Autodesk Inventor part; units mm, degrees
ref_plane "Work Plane2" through (-73.7, 7.425, 1.675) normal (-1, 0, 0) x (0, 0, 1)
ref_plane "Work Plane4" through (-27.2, 7.425, 1.675) normal (1, 0, 0) x (0, 1, 0)
ref_plane "Work Plane6" through (-32.2, 6.75, 1) normal (1, 0, 0) x (0, 1, 0)
ref_plane "Work Plane1" through (-24.5, 21.125, 15.375) normal (1, 0, 0) x (0, -1, 0)
sketch "Sketch1" plane through (-24.5, 21.125, 15.375) normal (1, 0, 0) x (0, -1, 0)
  line L0 (-16.375, 15.375) -> (19, 15.375)
  line L1 (19, 15.375) -> (19, -3.0564)
  line L2 (19, -3.0564) -> (-16.375, -3.0564)
  line L3 (-16.375, -3.0564) -> (-16.375, 15.375)
  circle A0 centre (1, 0) radius 5
  circle A1 centre (9, 0) radius 1.0564
  circle A2 centre (-7, 0) radius 1.0564
  circle A3 centre (1, 0) radius 5
  circle A4 centre (1, 0) radius 13.7
  line L4 (93.625, 18.375) -> (-16.375, 18.375)
  line L5 (-16.375, 18.375) -> (-16.375, 15.375)
  line L6 (93.625, 15.375) -> (-16.375, 15.375)
  line L7 (93.625, 18.375) -> (93.625, 15.375)
  point P0 (21.125, 15.375)
  point P1 (9, -1.0564)
  dimension "d5" = 2.1129
  dimension "d0" = 2
  dimension "d2" = 17.375
  dimension "d3" = 18
  dimension "d6" = 1.0564
extrude "Extrusion1" add sketch "Sketch1" along normal blind 2 and the other way blind 53.2 contours L0 L1 L2 A4 L3 | A4 L2 A0 | A0 L2 | A1 | A2 picked at (8.3146, 4.455) picked at (0.6453, -0.039)
sketch "Sketch2" plane through (-77.7, 21.125, 15.375) normal (-1, 0, 0) x (0, 0, 1)
  circle A0 centre (0, -1) radius 5
  line L0 (-1.5, 10) -> (1.5, 10)
  line L1 (1.5, 10) -> (1.5, 10.5)
  line L2 (1.5, 10.5) -> (-1.5, 10.5)
  line L3 (-1.5, 10.5) -> (-1.5, 10)
  line L4 (1.5, -12.5) -> (-1.5, -12.5)
  line L5 (-1.5, -12.5) -> (-1.5, -13)
  line L6 (-1.5, -13) -> (1.5, -13)
  line L7 (1.5, -13) -> (1.5, -12.5)
  line L8 (2, 9.5) -> (-2, 9.5)
  line L9 (-2, 9.5) -> (-2, 11)
  line L10 (-2, 11) -> (2, 11)
  line L11 (2, 11) -> (2, 9.5)
  line L12 (2, -13.5) -> (-2, -13.5)
  line L13 (-2, -13.5) -> (-2, -12)
  line L14 (-2, -12) -> (2, -12)
  line L15 (2, -12) -> (2, -13.5)
  circle A1 centre (0, -1) radius 5.2
  line L16 (3.0564, 16.375) -> (3.0564, -19)
  line L17 (2, 9.5) -> (3.0564, 9.5)
  line L18 (3.0564, 9.5) -> (3.0564, 12)
  line L19 (3.0564, 12) -> (2, 12)
  line L20 (2, 12) -> (2, 9.5)
  line L21 (2, -13.5) -> (3.0564, -13.5)
  line L22 (3.0564, -13.5) -> (3.0564, -11)
  line L23 (3.0564, -11) -> (2, -11)
  line L24 (2, -11) -> (2, -13.5)
  point P0 (-15.375, -21.125)
  point P1 (2, -11)
  point P2 (3.0564, -13.5)
  point P3 (3.0564, -11)
  point P4 (2, 12)
  point P5 (3.0564, 9.5)
  dimension "d11" = 0.5
  dimension "d12" = 0.5
  dimension "d13" = 0.2
ref_plane "Work Plane2" through (-73.7, 7.425, 1.675) normal (-1, 0, 0) x (0, 0, 1)
extrude "Extrusion2" cut sketch "Sketch2" against normal up to surface (4 mm away) contours A0 L16 | A0 L16 A1 | L16 A0 | A0 L16 A1 | L16 L21 L15 L24 L23 | L17 L11 L20 L19 L16 | L8 L9 L10 L11 | L12 L13 L14 L15 | L3 L2 L1 L0 | L7 L6 L5 L4
ref_plane "Work Plane3" through (-73.7, 21.125, 15.375) normal (-1, 0, 0) x (0, 1, 0)
sketch "Sketch3" plane through (-73.7, 21.125, 15.375) normal (-1, 0, 0) x (0, 1, 0)
  line L0 (10, 1.5) -> (10.5, 1.5)
  line L1 (10.5, 1.5) -> (10.5, -1.5)
  line L2 (10.5, -1.5) -> (10, -1.5)
  line L3 (10, -1.5) -> (10, 1.5)
  line L4 (-12.5, -1.5) -> (-13, -1.5)
  line L5 (-13, -1.5) -> (-13, 1.5)
  line L6 (-13, 1.5) -> (-12.5, 1.5)
  line L7 (-12.5, 1.5) -> (-12.5, -1.5)
  circle A0 centre (-1, 0) radius 5
  circle A1 centre (-1, 0) radius 13.7
  point P0 (-21.125, 15.375)
ref_plane "Work Plane4" through (-27.2, 7.425, 1.675) normal (1, 0, 0) x (0, 1, 0)
extrude "Extrusion3" cut sketch "Sketch3" against normal up to surface (46.5 mm away) contours L0 L1 L2 L3 | L4 L5 L6 L7 | A0 | A1
ref_plane "Work Plane5" through (-59.9, 21.125, 15.375) normal (-1, 0, 0) x (0, 1, 0)
sketch "Sketch4" plane through (-59.9, 21.125, 15.375) normal (-1, 0, 0) x (0, 1, 0)
  circle A0 centre (-1, 0) radius 14.375
  point P0 (-21.125, 15.375)
ref_plane "Work Plane6" through (-32.2, 6.75, 1) normal (1, 0, 0) x (0, 1, 0)
extrude "Extrusion4" cut sketch "Sketch4" against normal up to surface (27.7 mm away)
sketch "Sketch5" plane through (-22.5, 21.125, 15.375) normal (1, 0, 0) x (0, 0, -1)
  circle A0 centre (0, -9) radius 1.0564
  circle A1 centre (0, 7) radius 1.0564
  arc A2 (5.1468, 2.7666) -> (3.0755, 2.3394) centre (5.0543, -2.0206) ccw
  arc A3 (3.0755, 2.3394) -> (2.6716, 2.7917) centre (0, 0) ccw
  arc A4 (2.6716, 2.7917) -> (3.3299, 4.8016) centre (-1.4371, 5.2501) ccw
  arc A5 (3.3299, 4.8016) -> (2.5377, 5.2634) centre (0, 0) ccw
  arc A6 (2.5377, 5.2634) -> (1.113, 3.7003) centre (5.2767, 1.3362) ccw
  arc A7 (1.113, 3.7003) -> (0.5205, 3.8289) centre (0, 0) ccw
  arc A8 (0.5205, 3.8289) -> (-0.1284, 5.8419) centre (-4.2486, 3.4027) ccw
  arc A9 (-0.1284, 5.8419) -> (-1.0407, 5.7498) centre (0, 0) ccw
  arc A10 (-1.0407, 5.7498) -> (-1.2746, 3.6479) centre (3.4835, 4.1825) ccw
  arc A11 (-1.2746, 3.6479) -> (-1.8295, 3.4036) centre (0, 0) ccw
  arc A12 (-1.8295, 3.4036) -> (-3.5377, 4.6507) centre (-5.4372, 0.2556) ccw
  arc A13 (-3.5377, 4.6507) -> (-4.2216, 4.04) centre (0, 0) ccw
  arc A14 (-4.2216, 4.04) -> (-3.1753, 2.202) centre (0.3598, 5.4313) ccw
  arc A15 (-3.1753, 2.202) -> (-3.4807, 1.6782) centre (0, 0) ccw
  arc A16 (-3.4807, 1.6782) -> (-5.5956, 1.6831) centre (-4.549, -2.9892) ccw
  arc A17 (-5.5956, 1.6831) -> (-5.79, 0.787) centre (0, 0) ccw
  arc A18 (-5.79, 0.787) -> (-3.8632, -0.0849) centre (-2.9013, 4.6055) ccw
  arc A19 (-3.8632, -0.0849) -> (-3.8023, -0.6882) centre (0, 0) ccw
  arc A20 (-3.8023, -0.6882) -> (-5.5163, -1.9274) centre (-1.9232, -5.0921) ccw
  arc A21 (-5.5163, -1.9274) -> (-5.1468, -2.7666) centre (0, 0) ccw
  arc A22 (-5.1468, -2.7666) -> (-3.0755, -2.3394) centre (-5.0543, 2.0206) ccw
  arc A23 (-3.0755, -2.3394) -> (-2.6716, -2.7917) centre (0, 0) ccw
  arc A24 (-2.6716, -2.7917) -> (-3.3299, -4.8016) centre (1.4371, -5.2501) ccw
  arc A25 (-3.3299, -4.8016) -> (-2.5377, -5.2634) centre (0, 0) ccw
  arc A26 (-2.5377, -5.2634) -> (-1.113, -3.7003) centre (-5.2767, -1.3362) ccw
  arc A27 (-1.113, -3.7003) -> (-0.5205, -3.8289) centre (0, 0) ccw
  arc A28 (-0.5205, -3.8289) -> (0.1284, -5.8419) centre (4.2486, -3.4027) ccw
  arc A29 (0.1284, -5.8419) -> (1.0407, -5.7498) centre (0, 0) ccw
  arc A30 (1.0407, -5.7498) -> (1.2746, -3.6479) centre (-3.4835, -4.1825) ccw
  arc A31 (1.2746, -3.6479) -> (1.8295, -3.4036) centre (0, 0) ccw
  arc A32 (1.8295, -3.4036) -> (3.5377, -4.6507) centre (5.4372, -0.2556) ccw
  arc A33 (3.5377, -4.6507) -> (4.2216, -4.04) centre (0, 0) ccw
  arc A34 (4.2216, -4.04) -> (3.1753, -2.202) centre (-0.3598, -5.4313) ccw
  arc A35 (3.1753, -2.202) -> (3.4807, -1.6782) centre (0, 0) ccw
  arc A36 (3.4807, -1.6782) -> (5.5956, -1.6831) centre (4.549, 2.9892) ccw
  arc A37 (5.5956, -1.6831) -> (5.79, -0.787) centre (0, 0) ccw
  arc A38 (5.79, -0.787) -> (3.8632, 0.0849) centre (2.9013, -4.6055) ccw
  arc A39 (3.8632, 0.0849) -> (3.8023, 0.6882) centre (0, 0) ccw
  arc A40 (3.8023, 0.6882) -> (5.5163, 1.9274) centre (1.9232, 5.0921) ccw
  arc A41 (5.5163, 1.9274) -> (5.1468, 2.7666) centre (0, 0) ccw
  circle A42 centre (0, 0) radius 5.8433
  circle A43 centre (0, 0) radius 6.3433
  point P0 (15.375, -21.125)
  dimension "d20" = 0.5
extrude "Extrusion5" cut sketch "Sketch5" along normal mid plane 10 contours A0 | A1 A43 | A43 A1 | A1 A43 | A41 A40 A39 A38 A37 A36 A35 A34 A33 A32 A31 A30 A29 A28 A27 A26 A25 A24 A23 A22 A21 A20 A19 A18 A17 A16 A15 A14 A13 A12 A11 A10 A9 A8 A7 A6 A5 A4 A3 A2 | A2 A3 A4 A42 | A42 A38 A39 A40 | A6 A7 A8 A42 | A42 A34 A35 A36 | A10 A11 A12 A42 | A42 A30 A31 A32 | A14 A15 A16 A42 | A42 A26 A27 A28 | A18 A19 A20 A42 | A42 A22 A23 A24
sketch "Sketch6" plane through (-77.7, 37.5, 18.4314) normal (0, 0, 1) x (1, 0, 0)
  line L0 (50.5, -10.8166) -> (55.2, -10.8166)
  line L1 (55.2, 0) -> (55.2, -10.8166)
  line L2 (0, 0) -> (55.2, 0)
  line L3 (0, -4.375) -> (0, 0)
  line L4 (0, -4.375) -> (4, -4.375)
  line L5 (4, -30.7297) -> (4, -29.875)
  line L6 (4, -4.0203) -> (17.8, -4.0203)
  line L7 (17.8, -4.0203) -> (17.8, -3.3287)
  line L8 (17.8, -3.3287) -> (45.5, -3.3287)
  line L9 (45.5, -3.3287) -> (45.5, -4.0203)
  line L10 (45.5, -4.0203) -> (50.5, -4.0203)
  line L11 (50.5, -4.0203) -> (50.5, -10.8166)
  line L12 (55.2, -21.9334) -> (50.5, -21.9334)
  line L13 (50.5, -21.9334) -> (50.5, -30.7297)
  line L14 (50.5, -30.7297) -> (45.5, -30.7297)
  line L15 (45.5, -30.7297) -> (45.5, -31.4213)
  line L16 (45.5, -31.4213) -> (17.8, -31.4213)
  line L17 (17.8, -31.4213) -> (17.8, -30.7297)
  line L18 (4, -30.7297) -> (4, -29.875)
  line L19 (4, -29.875) -> (0, -29.875)
  line L20 (0, -35.375) -> (0, -29.875)
  line L21 (55.2, -35.375) -> (0, -35.375)
  line L22 (55.2, -21.9334) -> (55.2, -35.375)
  line L23 (50.5, -10.8166) -> (55.2, -10.8166)
  line L24 (55.2, 0) -> (55.2, -10.8166)
  line L25 (0, 0) -> (55.2, 0)
  line L26 (0, -4.375) -> (0, 0)
  line L27 (0, -4.375) -> (4, -4.375)
  line L28 (4, -4.375) -> (4, -4.0203)
  line L29 (4, -4.0203) -> (17.8, -4.0203)
  line L30 (45.5, -4.0203) -> (50.5, -4.0203)
  line L31 (50.5, -4.0203) -> (50.5, -10.8166)
  line L32 (17.8, -4.0203) -> (17.8, -3.3287)
  line L33 (17.8, -3.3287) -> (45.5, -3.3287)
  line L34 (45.5, -3.3287) -> (45.5, -4.0203)
  line L35 (17.8, -30.7297) -> (4, -30.7297)
  line L36 (4, -27.375) -> (4, -21.5819)
  line L37 (4, -21.5819) -> (0, -21.5819)
  line L38 (0, -27.375) -> (0, -21.5819)
  line L39 (0, -27.375) -> (4, -27.375)
  line L40 (4, -13.1681) -> (4, -6.875)
  line L41 (4, -6.875) -> (0, -6.875)
  line L42 (0, -13.1681) -> (0, -6.875)
  line L43 (0, -13.1681) -> (4, -13.1681)
  line L44 (4, -27.375) -> (4, -21.5819)
  line L45 (4, -21.5819) -> (0, -21.5819)
  line L46 (0, -27.375) -> (0, -21.5819)
  line L47 (0, -27.375) -> (4, -27.375)
  line L48 (4, -13.1681) -> (4, -6.875)
  line L49 (4, -6.875) -> (0, -6.875)
  line L50 (0, -13.1681) -> (0, -6.875)
  line L51 (0, -13.1681) -> (4, -13.1681)
  line L52 (55.2, -21.9334) -> (50.5, -21.9334)
  line L53 (50.5, -21.9334) -> (50.5, -30.7297)
  line L54 (50.5, -30.7297) -> (45.5, -30.7297)
  line L55 (45.5, -30.7297) -> (45.5, -31.4213)
  line L56 (45.5, -31.4213) -> (17.8, -31.4213)
  line L57 (17.8, -31.4213) -> (17.8, -30.7297)
  line L58 (17.8, -30.7297) -> (4, -30.7297)
  line L59 (4, -29.875) -> (0, -29.875)
  line L60 (0, -35.375) -> (0, -29.875)
  line L61 (55.2, -35.375) -> (0, -35.375)
  line L62 (55.2, -21.9334) -> (55.2, -35.375)
  line L63 (4, -4.375) -> (4, -4.0203)
  point P0 (77.7, -37.5)
  point P1 (2, -2)
  point P2 (53.2, -2)
  point P3 (53.2, -33.375)
  point P4 (2, -33.375)
  dimension "d23" = 2
  dimension "d24" = 2
  dimension "d25" = 2
  dimension "d26" = 2
  dimension "d27" = 2
  dimension "d28" = 2
  dimension "d29" = 2
  dimension "d30" = 2
properties part number "right_motor_mount"
Here's how the part is built. I have some questions about the finished solid (model axes, mm). A direction names the side the tool comes from. Round coordinates to 2 decimals unless told otherwise and drop trailing zeros. Order: outer loops, then holes, each group sorted by start corner. A loop starts at its lowest first (then second) coordinate and runs counter-clockwise, first axis right, second up. Notation, with made-up numbers: M 68.25,58.25 L 127.25,58.25 A30 cw 127.25,93.25 Z; hole C -40,-0.75 d8. An arc over 180 degrees is marked long. One line per question, with ' | ' between items.
1) I'm going to push flat-ended pins straight in: pin 1 Ø3.5 at (y, z) = (28.125, 15.375) entering from +X; pin 2 Ø5 at (y, z) = (21.5, 12.5) entering from +X; pin 3 Ø1.5 at (x, y) = (-65.5, 31.5) entering from +Z; pin 4 Ø0.8 at (x, y) = (-76.5, 9.5) entering from +Z (3 decimals). Where does each tip first touch, or does it pass through?
Checked values:
pin 1: stops at x = -22.5 | pin 2: stops at x = -73.7 | pin 3: stops at z = 9 | pin 4: stops at z = 17.375
2) Imagine slicing it at A-A, the plane z = 10.75. Write out the boundary of the cut face in (x, y) (3 decimals).
Checked values:
outline: M -77.7,2.125 L -22.5,2.125 L -22.5,16.784 L -27.2,16.784 L -27.2,7.229 L -32.2,7.229 L -32.2,6.514 L -59.9,6.514 L -59.9,7.229 L -73.7,7.229 L -73.7,17.748 L -77.7,17.748 Z; M -77.7,22.502 L -73.7,22.502 L -73.7,33.021 L -59.9,33.021 L -59.9,33.736 L -32.2,33.736 L -32.2,33.021 L -27.2,33.021 L -27.2,25.466 L -22.5,25.466 L -22.5,37.5 L -77.7,37.5 Z
3) We'd pull the mould along X, two halves only. Please class faces 6 (the flat face through (-22.5, 20, 7)), 7 (the cylindrical face through (-24.8, 19, 9.4)), 8 (the cylindrical face through (-29.74, 20.47, 1.68)): released by +X, released by -X, zero draft, split by the parting line, or undercut.
Checked values:
face 6: released by +X | face 7: zero draft | face 8: undercut
4) I need wall thicknesses on line 1 (X direction, y = 16.5, z = 3.5); line 2 (X direction, y = 26, z = 17.25); line 3 (Y direction, x = -58.5, z = 16) (3 decimals). Which ranges of each line are inside material? Lowest first, please.
Checked values:
line 1: x = -77.7 to -73.7, -27.2 to -22.5 | line 2: x = -77.7 to -73.7 | line 3: y = 2.125 to 5.764, 34.486 to 37.5
5) Imagine slicing it at D-D, the plane x = -31.5. Write out the boundary of the cut face in (y, z) (3 decimals).
Checked values:
outline: M 2.125,0 L 37.5,0 L 37.5,18.431 L 33.48,18.431 A13.7 cw long 6.77,18.431 L 2.125,18.431 Z
6) Imagine slicing it at B-B, the plane z = 7.5. Write out the boundary of the cut face in (x, y) (3 decimals).
Checked values:
outline: M -77.7,2.125 L -22.5,2.125 L -22.5,37.5 L -77.7,37.5 Z; hole M -73.7,8.915 L -59.9,8.915 L -59.9,8.099 L -32.2,8.099 L -32.2,8.915 L -27.2,8.915 L -27.2,31.335 L -32.2,31.335 L -32.2,32.151 L -59.9,32.151 L -59.9,31.335 L -73.7,31.335 Z
7) Imagine slicing it at C-C, the plane y = 16.5. Write out the boundary of the cut face in (x, z), plus the area to 3 significant figures.
Checked values:
outline: M -77.7,0 L -22.5,0 L -22.5,11.03 L -27.2,11.03 L -27.2,2.16 L -32.2,2.16 L -32.2,1.46 L -59.9,1.46 L -59.9,2.16 L -73.7,2.16 L -73.7,11.65 L -77.7,11.65 Z | area: 180 mm²
8) On a 3-axis mill with a long thin cutter (end or side, diameter ignored), from which of +Z, -Z, +X, -X, +Y, -Y can I reach the whole of each face in a straight line? I mean faces 1 (the flat face through (-76, 8, 13.375)), 2 (the cylindrical face through (-75.728, 20.285, 10.177)), 3 (the cylindrical face through (-24.817, 11.188, 14.888)), 4 (the cylindrical face through (-46, 20, 1)), 5 (the flat face through (-76, 13, 18.431)). Say none if no direction works.
Checked values:
face 1: +Z, -X | face 2: +X, -X | face 3: +X | face 4: none | face 5: +Z, +X, -X, +Y, -Y
